Check sheet for the modelled part. Datum: model origin and axes. Units: mm. Coordinates: 2 decimals unless noted, no trailing zeros. Order: outer loops, then holes, each group sorted by start corner. A loop starts at its lowest first (then second) coordinate and runs counter-clockwise, first axis right, second up.
1. Draft check along X on faces 1 (the flat face through (9, 1, 0)), 2 (the flat face through (-8.724, 0, 4)), 3 (the cylindrical face through (20.011, 1.687, 4.056)). Enter one of: released by +X, released by -X, zero draft, split by the parting line, or undercut.
2. Cross-section at D-D (y = -0.25). Enter the section's corners in (x, z), then the cut area to 3 significant figures.
3. Gauge pin test, flat ends, axial feed: pin 1 Ø3 at (x, y) = (15, 0.5) entering from -Z; pin 2 Ø1.8 at (x, y) = (21.28, 0.88) entering from -Z. Record the tip position at first contact, or that the pin passes through.
4. Cross-section at A-A (z = 4.5). Enter the section's corners in (x, y).
5. Thickness scan on line 1 (X direction, y = 1.75, z = 7); line 2 (X direction, y = 2.25, z = 7.75); line 3 (X direction, y = 4.75, z = 4.5). Record the ranges inside material, lowest first.
6. Cross-section at C-C (z = 6.5). Enter the section's corners in (x, y).
7. Cross-section at B-B (y = 1.25). Enter the section's corners in (x, z).
Autodesk Inventor part; units mm, degrees
ref_plane "YZ Plane" through (0, 0, 0) normal (1, 0, 0) x (0, 1, 0)
ref_plane "XZ Plane" through (0, 0, 0) normal (0, 1, 0) x (-1, 0, 0)
ref_plane "XY Plane" through (0, 0, 0) normal (0, 0, 1) x (1, 0, 0)
sketch "Sketch1" plane through (0, 0, 0) normal (0, 0, 1) x (1, 0, 0)
  line L0 (-8.7244, 5.8803) -> (27.2756, 5.8803)
  line L1 (27.2756, 5.8803) -> (27.2756, -4.1197)
  line L2 (27.2756, -4.1197) -> (-8.7244, -4.1197)
  line L3 (-8.7244, -4.1197) -> (-8.7244, 5.8803)
  point P0 (0, 0)
  point P1 (-2.7244, 0.8803)
  point P2 (21.2756, 0.8803)
  dimension "d0" = 36
  dimension "d1" = 24
  dimension "d2" = 6
  dimension "d3" = 10
  dimension "d4" = 5
extrude "Extrusion1" add sketch "Sketch1" along normal blind 8
hole "Hole1" at (-2.7244, 0.8803, 0) at (21.2756, 0.8803, 0) direction (0, 0, 1) diameter 3 end through all
sketch "Sketch2" plane through (-8.7244, 5.8803, 0) normal (0, 1, 0) x (1, 0, 0)
  line L0 (0, 0) -> (36, 0)
  line L1 (0, 0) -> (0, -8)
  line L2 (36, -8) -> (0, -8)
  line L3 (36, 0) -> (36, -8)
  line L4 (0, -8) -> (36, -8)
  circle A0 centre (18, -8.3) radius 6
  point P0 (8.7244, 0)
  dimension "d15" = 36
  dimension "d22" = 12
  dimension "d23" = 18
  dimension "d24" = 0.3
extrude "Extrusion2" cut sketch "Sketch2" against normal through all contours A0 L2 | L2 A0
chamfer "Chamfer1" distance 2 angle 45 2 edges at (27.2756, 5.8803, 4) (-8.7244, 5.8803, 4)
equation "\"d23\" = 0.5 * d15"
properties part number "3DP_PLA_X_axis_carriage_laser_mount_clamp" material "ABS Plastic"
Data:
1. face 1: zero draft
1. face 2: released by -X
1. face 3: undercut
2. outline: (-8.72, 0) - (-3.71, 0) - (-3.71, 8) - (-8.72, 8) - close; (-1.74, 0) - (20.29, 0) - (20.29, 8) - (15.27, 8) arc R6 cw to (3.28, 8) - (-1.74, 8) - close; (22.26, 0) - (27.28, 0) - (27.28, 8) - (22.26, 8) - close
2. area: 203 mm2
3. pin 1: stops at z = 0
3. pin 2: passes through
4. outline: (-8.72, -4.12) - (4.63, -4.12) - (4.63, 5.88) - (-6.72, 5.88) - (-8.72, 3.88) - close; (13.92, -4.12) - (27.28, -4.12) - (27.28, 3.88) - (25.28, 5.88) - (13.92, 5.88) - close; hole circle Ø3 at (-2.72, 0.88); hole circle Ø3 at (21.28, 0.88)
5. line 1: x = -8.72 to -3.95, -1.5 to 3.42, 15.13 to 20.05, 22.5 to 27.28
5. line 2: x = -8.72 to -3.34, -2.11 to 3.3, 15.25 to 20.66, 21.89 to 27.28
5. line 3: x = -7.85 to 4.63, 13.92 to 26.41
6. outline: (-8.72, -4.12) - (3.55, -4.12) - (3.55, 5.88) - (-6.72, 5.88) - (-8.72, 3.88) - close; (15, -4.12) - (27.28, -4.12) - (27.28, 3.88) - (25.28, 5.88) - (15, 5.88) - close; hole circle Ø3 at (-2.72, 0.88); hole circle Ø3 at (21.28, 0.88)
7. outline: (-8.72, 0) - (-4.18, 0) - (-4.18, 8) - (-8.72, 8) - close; (-1.27, 0) - (19.82, 0) - (19.82, 8) - (15.27, 8) arc R6 cw to (3.28, 8) - (-1.27, 8) - close; (22.73, 0) - (27.28, 0) - (27.28, 8) - (22.73, 8) - close
